Autodesk Inventor part; units mm, degrees
ref_plane "YZ Plane" through (0, 0, 0) normal (1, 0, 0) x (0, 1, 0)
ref_plane "XZ Plane" through (0, 0, 0) normal (0, 1, 0) x (-1, 0, 0)
ref_plane "XY Plane" through (0, 0, 0) normal (0, 0, 1) x (1, 0, 0)
sketch "Szkic1" plane through (0, 0, 0) normal (0, 0, 1) x (1, 0, 0)
  line L0 (-15, -8.5) -> (15, -8.5)
  line L1 (15, -8.5) -> (15, 4.5)
  line L2 (11, 8.5) -> (-11, 8.5)
  line L3 (-15, 4.5) -> (-15, -8.5)
  line L4 (-15, -8.5) -> (15, 8.5) construction
  line L5 (15, -8.5) -> (-15, 8.5) construction
  line L6 (-13, 6.5) -> (13, 6.5)
  line L7 (13, 6.5) -> (13, -6.5)
  line L8 (13, -6.5) -> (-13, -6.5)
  line L9 (-13, -6.5) -> (-13, 6.5)
  line L10 (-5.5, -6.5) -> (5.5, -6.5)
  line L11 (5.5, -6.5) -> (5.5, 6.5)
  line L12 (5.5, 6.5) -> (-5.5, 6.5)
  line L13 (-5.5, 6.5) -> (-5.5, -6.5)
  line L14 (-5.5, -6.5) -> (5.5, 6.5) construction
  line L15 (5.5, -6.5) -> (-5.5, 6.5) construction
  line L16 (-5.5, -6.5) -> (-5.5, -8.5)
  line L17 (5.5, -6.5) -> (5.5, -8.5)
  line L18 (-11, 8.5) -> (-15, 4.5)
  line L19 (11, 8.5) -> (15, 4.5)
  point P0 (0, 0)
  dimension "d0" = 30
  dimension "d1" = 17
  dimension "d2" = 2
  dimension "d3" = 11
  dimension "d4" = 4
  dimension "d5" = 4
  dimension "d6" = 4
  dimension "d7" = 4
extrude "Wyciągnięcie proste1" add sketch "Szkic1" along normal blind 10 contours L3 L18 L9 L8 L16 L0 | L17 L8 L7 L19 L1 L0 | L8 L9 L6 L13 | L18 L2 L19 L6 | L11 L6 L7 L8
sketch "Szkic2" plane through (0, 0, 0) normal (0, 0, -1) x (-1, 0, 0)
  line L0 (5.5, 6.5) -> (-5.5, 6.5)
  line L1 (5.5, -8.5) -> (5.5, 6.5)
  line L2 (15, -8.5) -> (5.5, -8.5)
  line L3 (15, 4.5) -> (15, -8.5)
  line L4 (11, 8.5) -> (15, 4.5)
  line L5 (-11, 8.5) -> (11, 8.5)
  line L6 (-15, 4.5) -> (-11, 8.5)
  line L7 (-15, -8.5) -> (-15, 4.5)
  line L8 (-5.5, -8.5) -> (-15, -8.5)
  line L9 (-5.5, 6.5) -> (-5.5, -8.5)
  line L10 (-5.5, -8.5) -> (5.5, -8.5)
  point P0 (0, 0)
extrude "Wyciągnięcie proste2" add sketch "Szkic2" along normal blind 10
sketch "Szkic3" plane through (0, 0, -10) normal (0, 0, -1) x (-1, 0, 0)
  line L0 (15, -8.5) -> (15, 4.5)
  line L1 (15, 4.5) -> (11, 8.5)
  line L2 (11, 8.5) -> (-11, 8.5)
  line L3 (-11, 8.5) -> (-15, 4.5)
  line L4 (-15, 4.5) -> (-15, -8.5)
  line L5 (-15, -8.5) -> (15, -8.5)
  line L6 (10.1716, 6.5) -> (13, 3.6716)
  line L7 (13, 3.6716) -> (13, -6.5)
  line L8 (13, -6.5) -> (-13, -6.5)
  line L9 (-13, -6.5) -> (-13, 3.6716)
  line L10 (-13, 3.6716) -> (-10.1716, 6.5)
  line L11 (-10.1716, 6.5) -> (10.1716, 6.5)
  line L12 (-13, -6.5) -> (-13, -8.5)
  line L13 (13, -6.5) -> (13, -8.5)
  point P0 (0, 0)
  dimension "d12" = 2
extrude "Wyciągnięcie proste3" cut sketch "Szkic3" against normal blind 7 contours L5 L12 L8 L13 | L8 L9 L10 L11 L6 L7
sketch "Szkic4" plane through (15, -8.5, 10) normal (1, 0, 0) x (0, 0, -1)
  line L0 (20, 0) -> (0, 0)
  line L1 (20, 0) -> (18, 0)
  line L2 (18, 0) -> (20, 12.8915)
  line L3 (20, 12.8915) -> (20, 0)
  point P0 (10, 8.5)
  dimension "d15" = 2
extrude "Wyciągnięcie proste4" cut sketch "Szkic4" against normal through all
sketch "Szkic6" plane through (0, 0, -3) normal (0, 0, -1) x (-1, 0, 0)
  line L0 (-11, 4.5) -> (11, 4.5)
  line L1 (11, 4.5) -> (11, -17.5)
  line L2 (11, -17.5) -> (-11, -17.5)
  line L3 (-11, -17.5) -> (-11, 4.5)
  line L4 (13, -8.5) -> (-13, -8.5)
  line L5 (-11, 4.5) -> (11, 4.5)
  line L6 (11, 4.5) -> (11, -8.5)
  line L7 (11, -8.5) -> (-11, -8.5)
  line L8 (-11, -8.5) -> (-11, 4.5)
  point P0 (0, 0)
  dimension "d18" = 22
  dimension "d19" = 22
extrude "Wyciągnięcie proste5" add sketch "Szkic6" along normal blind 40 contours L0 L1 L4 L3
fillet "Zaokrąglenie1" radius 2 4 edges at (11, 4.5, -23) (11, -8.5, -23) (-11, -8.5, -23) (-11, 4.5, -23)
sketch "Szkic7" plane through (0, 0, -43) normal (0, 0, -1) x (-1, 0, 0)
  line L0 (11, -6.5) -> (11, 2.5)
  arc A0 (11, 2.5) -> (9, 4.5) centre (9, 2.5) ccw
  line L1 (9, 4.5) -> (-9, 4.5)
  arc A1 (-9, 4.5) -> (-11, 2.5) centre (-9, 2.5) ccw
  line L2 (-11, 2.5) -> (-11, -6.5)
  arc A2 (-11, -6.5) -> (-9, -8.5) centre (-9, -6.5) ccw
  line L3 (-9, -8.5) -> (9, -8.5)
  arc A3 (9, -8.5) -> (11, -6.5) centre (9, -6.5) ccw
  line L4 (11, -6.5) -> (11, 2.5)
  line L5 (-7, 2.5) -> (7, 2.5)
  line L6 (9, 0.5) -> (9, -4.5)
  line L7 (7, -6.5) -> (-7, -6.5)
  line L8 (-9, -4.5) -> (-9, 0.5)
  arc A4 (-7, 2.5) -> (-9, 0.5) centre (-7, 0.5) ccw
  arc A5 (-9, -4.5) -> (-7, -6.5) centre (-7, -4.5) ccw
  arc A6 (7, -6.5) -> (9, -4.5) centre (7, -4.5) ccw
  arc A7 (9, 0.5) -> (7, 2.5) centre (7, 0.5) ccw
  point P0 (0, 0)
  dimension "d23" = 2
  dimension "d24" = 2
extrude "Wyciągnięcie proste6" cut sketch "Szkic7" against normal blind 25 contours L5 A7 L6 A6 L7 A5 L8 A4
equation "\"d5\" = d4"
equation "\"d6\" = d4"
equation "\"d7\" = d6"
properties part number "gunv1"
Input: part model. Units: mm. Frame: model coordinates. A direction names the side the tool comes from. Round coordinates to 2 decimals unless told otherwise and drop trailing zeros. Loops run counter-clockwise (first coordinate to the right, second up) from the corner with the lowest first, then second, coordinate; pieces in that order, holes last. Notation, with made-up numbers: (50.5, 28.5) - (72.5, 28.5) arc R17 ccw to (72.5, 37.5) - close; hole circle Ø11 at (12, -18). An arc over 180 degrees is marked (long way). One line per item, written item: value. Start each with the question number.
(1) Draft query along Y for faces 4 (the flat face through (-13, -2, -6)), 5 (the flat face through (13.961, -2.144, -8.986)), 6 (the flat face through (11.606, 5.066, -6.549)). Return one class per face: +Y half, -Y half, draft (parallel to the pull), parting line (faces both ways), or undercut.
(2) Section D-D, the plane y = 5.5. Return loops of the section in (x, z), plus the area to 3 significant figures.
(3) Section B-B, the plane x = 4. Return loops of the section in (y, z), plus the area to 3 significant figures.
(4) Access query for faces 1 (the flat face through (13, -2, -6)), 2 (the flat face through (-5.5, -1, 5)), 3 (the flat face through (9, -2, -31)). Directions: +Z, -Z, +X, -X, +Y, -Y. A direction counts if a zero-diameter tool reaches every point of the face in a straight line with its end or side. Return the directions, or none.
(5) Section A-A, the plane z = -31. Return loops of the section in (x, y).
(6) Ray query, line 1 (Y direction, x = -3.5, z = -8); line 2 (X direction, y = 0, z = -38); line 3 (Y direction, x = 2, z = -34.5). Return the intervals inside material, ascending. Write a range as [from, to].
(7) Section C-C, the plane y = -0.5. Return loops of the section in (x, z), plus the area to 3 significant figures.
(8) Contact query for flat-ended pins moving along their axis: P1, Ø5.5, axis at x = -4, z = -28.5, coming from the +Y side; P2, Ø4.5, axis at y = -2.5, z = -23.5, coming from the +X side; P3, Ø1.5, axis at x = 1.5, y = -4, coming from the -Z side. Output: stop coordinate, or through.
Results below:
1. face 4: draft
1. face 5: -Y half
1. face 6: undercut
2. outline: (-14, -10) - (-11.17, -10) - (-11.17, -3) - (11.17, -3) - (11.17, -10) - (14, -10) - (14, 10) - (5.5, 10) - (5.5, 0) - (-5.5, 0) - (-5.5, 10) - (-14, 10) - close
2. area: 294 mm^2
3. outline: (-8.5, -43) - (-6.5, -43) - (-6.5, -18) - (2.5, -18) - (2.5, -43) - (4.5, -43) - (4.5, -3) - (6.5, -3) - (6.5, -10) - (8.5, -10) - (8.5, 10) - (6.5, 10) - (6.5, 0) - (-8.5, 0) - close
3. area: 380 mm^2
4. face 1: -Z, -Y
4. face 2: +Z, -Y
4. face 3: -Z
5. outline: (-11, -6.5) arc R2 ccw to (-9, -8.5) - (9, -8.5) arc R2 ccw to (11, -6.5) - (11, 2.5) arc R2 ccw to (9, 4.5) - (-9, 4.5) arc R2 ccw to (-11, 2.5) - close; hole (-9, -4.5) arc R2 ccw to (-7, -6.5) - (7, -6.5) arc R2 ccw to (9, -4.5) - (9, 0.5) arc R2 ccw to (7, 2.5) - (-7, 2.5) arc R2 ccw to (-9, 0.5) - close
6. line 1: [-8.5, 4.5], [6.5, 8.5]
6. line 2: [-11, -9], [9, 11]
6. line 3: [-8.5, -6.5], [2.5, 4.5]
7. outline: (-15, -9.24) - (-13, -9.24) - (-13, -3) - (-11, -3) - (-11, -43) - (-9, -43) - (-9, -18) - (9, -18) - (9, -43) - (11, -43) - (11, -3) - (13, -3) - (13, -9.24) - (15, -9.24) - (15, 10) - (5.5, 10) - (5.5, 0) - (-5.5, 0) - (-5.5, 10) - (-15, 10) - close
7. area: 735 mm^2
8. P1: y = 4.5
8. P2: x = 11
8. P3: z = -18
